For this review, use the dimensioned drawing (mm, ordinates from the lowest corner) and the shaded views. A direction names the side the tool comes from. Coordinates: 2 decimals unless noted, no trailing zeros. Loops run counter-clockwise (first coordinate to the right, second up) from the corner with the lowest first, then second, coordinate; pieces in that order, holes last. Notation, with made-up numbers: M -39.5,1 L -0.5,1 A32 cw -0.5,38 Z; hole C 59,-10.75 d9. An arc over 180 degrees is marked long. Write item = value, one per line.
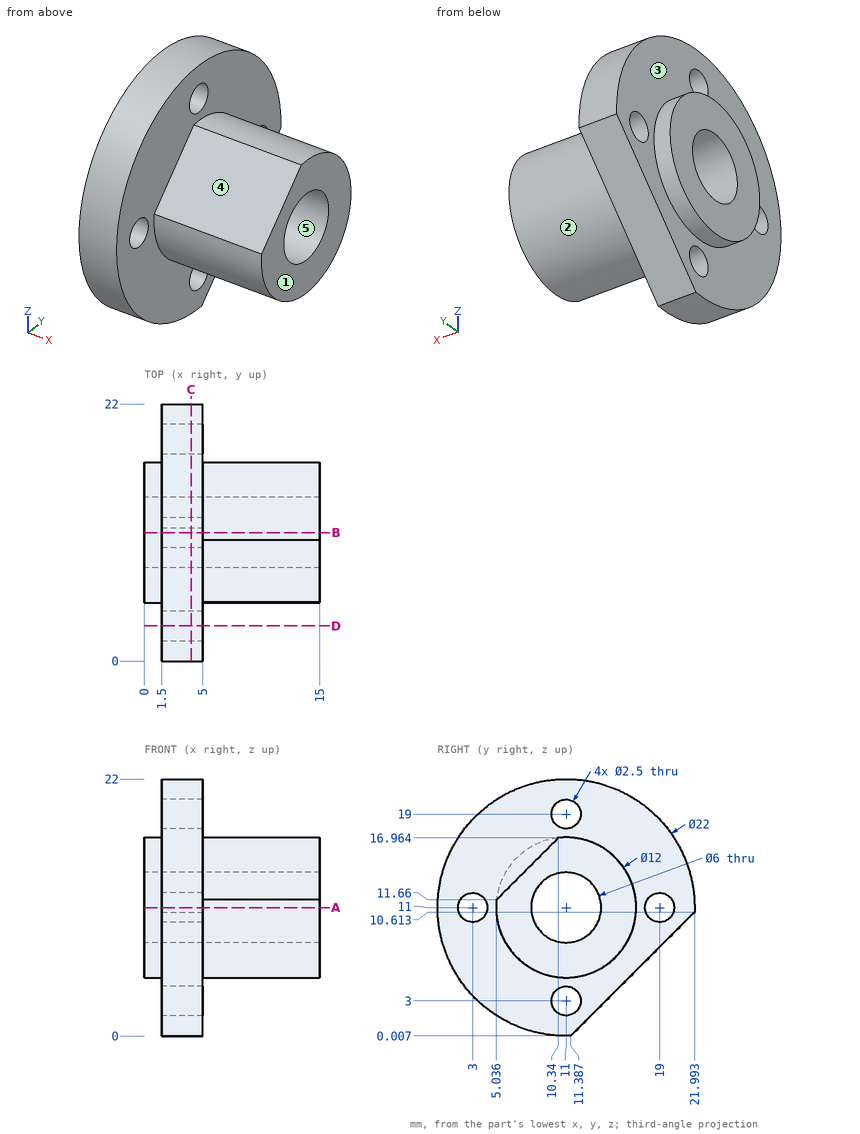
Q1. For pin 1 Ø6.5 at (y, z) = (11, 9) entering from +X; pin 2 Ø2 at (x, y) = (4, 9) entering from +Z (1 decimal); pin 3 Ø4 at (y, z) = (4.5, 16) entering from -X; pin 4 Ø1 at (x, z) = (7.5, 7.5) entering from -Y (1 decimal), all flat-tipped, find the tip position at first contact; note any pin that passes through.
Solved:
pin_1 = 15
pin_2 = 22
pin_3 = 1.5
pin_4 = 5.8
Q2. Machinability: for the marked faces 1, 2, 3, 4 and 5, which of the approach directions +Z, -Z, +X, -X, +Y, -Y give a long, thin tool a straight path to every point of the face, cutting with its end or side? Answer none if there is none.
Solved:
face_1 = +Z, -Z, +X, +Y, -Y
face_2 = +X
face_3 = -X
face_4 = +Z, +X, -Y
face_5 = +X, -X
Q3. Add section D-D (y = 3). Write out the cut boundary in (x, z).
Solved:
outline = M 1.5,3.45 L 5,3.45 L 5,9.75 L 1.5,9.75 Z; M 1.5,12.25 L 5,12.25 L 5,18.55 L 1.5,18.55 Z
Q4. Add section C-C (x = 4). Write out the cut boundary in (y, z), and give its area (3 significant figures).
Solved:
outline = M 11.39,0.01 L 21.99,10.61 A11 ccw long Z; hole C 3,11 d2.5; hole C 11,11 d6; hole C 11,3 d2.5; hole C 11,19 d2.5; hole C 19,11 d2.5
area = 302 mm²
Q5. Add section A-A (z = 11). Write out the cut boundary in (x, y).
Solved:
outline = M 0,5 L 1.5,5 L 1.5,4.25 L 5,4.25 L 5,5 L 15,5 L 15,8 L 0,8 Z; M 0,14 L 15,14 L 15,17 L 5,17 L 5,17.75 L 1.5,17.75 L 1.5,17 L 0,17 Z; M 1.5,0 L 5,0 L 5,1.75 L 1.5,1.75 Z; M 1.5,20.25 L 5,20.25 L 5,22 L 1.5,22 Z
Q6. For line 1 along Z through (x, y) = (3.95, 11); line 2 along Z through (x, y) = (7.5, 11); line 3 along Z through (x, y) = (3.35, 3), list the stretches that pass through material, from the lowest coordinate up.
Solved:
line_1 = 0 to 1.75, 4.25 to 8, 14 to 17.75, 20.25 to 22
line_2 = 5 to 8, 14 to 17
line_3 = 3.45 to 9.75, 12.25 to 18.55
